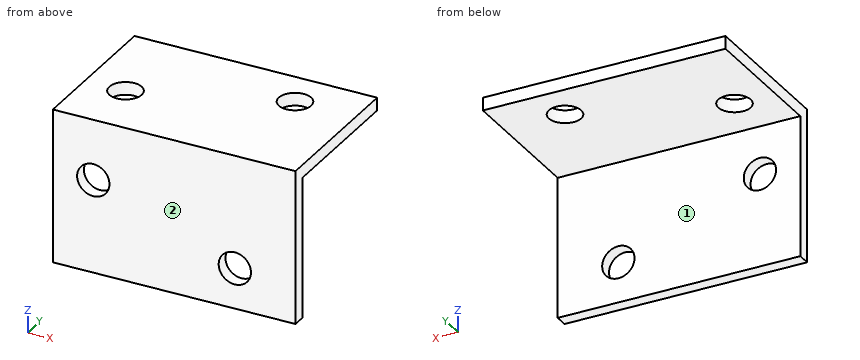
from build123d import *

# Parameters (mm, degrees)
SKETCH1_W           = 60
SKETCH1_H           = 38
BOSS_EXTRUDE1_DEPTH = 3.175
SKETCH2_W           = 60
SKETCH2_H           = 3.175
BOSS_EXTRUDE2_DEPTH = 34.825
SKETCH3_R           = 4
CUT_EXTRUDE1_DEPTH  = 80.099814317
SKETCH4_R           = 4
CUT_EXTRUDE2_DEPTH  = 78.624488726


with BuildPart() as part:
    # Sketch1 → Boss-Extrude1 (new body)
    with BuildSketch(Plane.XY):
        with Locations((30, 19)):
            Rectangle(SKETCH1_W, SKETCH1_H)
    extrude(amount=BOSS_EXTRUDE1_DEPTH)

    # Sketch2 → Boss-Extrude2 (add)
    with BuildSketch(Plane(origin=(0, 0, 0), x_dir=(-1, 0, 0), z_dir=(0, 0, -1))):
        with Locations((-30, 1.5875)):
            Rectangle(SKETCH2_W, SKETCH2_H)
    extrude(amount=BOSS_EXTRUDE2_DEPTH)

    # Sketch3 → Cut-Extrude1 (cut, through all)
    with BuildSketch(Plane(origin=(0, 0, 0), x_dir=(-1, 0, 0), z_dir=(0, 0, -1))):
        with Locations((-45, 28)):
            Circle(SKETCH3_R)
        with Locations((-10, 15)):
            Circle(SKETCH3_R)
    extrude(amount=-CUT_EXTRUDE1_DEPTH, mode=Mode.SUBTRACT)

    # Sketch4 → Cut-Extrude2 (cut, through all)
    with BuildSketch(Plane(origin=(0, 3.175, 0), x_dir=(1, 0, 0), z_dir=(0, 1, 0))):
        with Locations(Location((45, 24.825, 0), (0, 0, 180))):
            Circle(SKETCH4_R)
        with Locations(Location((10, 11.825, 0), (0, 0, 180))):
            Circle(SKETCH4_R)
    extrude(amount=-CUT_EXTRUDE2_DEPTH, mode=Mode.SUBTRACT)


solid = part.part
Part model, mm, in its own coordinate system. Face numbers are marked on the shaded views. A direction names the side the tool comes from. Round coordinates to 2 decimals unless told otherwise and drop trailing zeros. Order: outer loops, then holes, each group sorted by start corner. A loop starts at its lowest first (then second) coordinate and runs counter-clockwise, first axis right, second up. Notation, with made-up numbers: (-8.5, 83.25) -> (15.5, 83.25) arc R8 cw to (15.5, 90.25) -> close; hole circle Ø6 at (41.5, 43.5). An arc over 180 degrees is marked (long way). Put each result on its own line as item: value.
Q1. Band-saw the part on D-D (x = 39). Give the cut face in (y, z) (3 decimals), and give its area (3 significant figures).
From the geometry:
outline: (0, -34.825) -> (3.175, -34.825) -> (3.175, 0) -> (38, 0) -> (38, 3.175) -> (0, 3.175) -> close
area: 231 mm2
Q2. Pin check, flat tips, straight feed: pin 1 Ø1.5 at (x, z) = (19.5, -30) entering from +Y (3 decimals); pin 2 Ø10 at (x, z) = (29, -9) entering from -Y; pin 3 Ø10.5 at (x, y) = (39, 26.5) entering from -Z; pin 4 Ø6 at (y, z) = (29, -5) entering from +X. Stop position of each tip, or through.
From the geometry:
pin 1: stops at y = 3.175
pin 2: stops at y = 0
pin 3: stops at z = 0
pin 4: passes through
Q3. Band-saw the part on C-C (z = -10). Give the cut face in (x, y) (3 decimals).
From the geometry:
outline: (0, 0) -> (6.441, 0) -> (6.441, 3.175) -> (0, 3.175) -> close; (13.559, 0) -> (60, 0) -> (60, 3.175) -> (13.559, 3.175) -> close
Q4. Band-saw the part on A-A (y = 28). Give the cut face in (x, z) (3 decimals), and give its area (3 significant figures).
From the geometry:
outline: (0, 0) -> (41, 0) -> (41, 3.175) -> (0, 3.175) -> close; (49, 0) -> (60, 0) -> (60, 3.175) -> (49, 3.175) -> close
area: 165 mm2
Q5. Tool access for the marked faces 1 and 2: list every direction of +Z, -Z, +X, -X, +Y, -Y with a clear straight run to the whole face (end or side of a thin tool).
From the geometry:
face 1: -Z, +X, -X, +Y
face 2: +Z, -Z, +X, -X, -Y
Q6. Wall check: line 1 (Y direction, x = 45, z = 2.5); line 2 (Y direction, x = 10, z = 1); line 3 (Z direction, x = 10, y = 1.75) (3 decimals). Give the ranges that are in metal, low to high. Write a range as [from, to].
From the geometry:
line 1: y = [0, 24], [32, 38]
line 2: y = [0, 11], [19, 38]
line 3: z = [-34.825, -15.825], [-7.825, 3.175]
Q7. Band-saw the part on B-B (x = 10). Give the cut face in (y, z) (3 decimals).
From the geometry:
outline: (0, -34.825) -> (3.175, -34.825) -> (3.175, -15.825) -> (0, -15.825) -> close; (0, -7.825) -> (3.175, -7.825) -> (3.175, 0) -> (11, 0) -> (11, 3.175) -> (0, 3.175) -> close; (19, 0) -> (38, 0) -> (38, 3.175) -> (19, 3.175) -> close
